Autodesk Fusion 360 part; units mm, degrees
sketch "Skizze1" plane through (0, 0, 0) normal (0, 1, 0) x (1, 0, 0)
  circle A0 centre (0, 0) radius 71.7
  circle A1 centre (0, 0) radius 68.7
  circle A2 centre (0, 0) radius 25
  circle A3 centre (0, 44) radius 13.5
  circle A4 centre (-38.1051, 22) radius 13.5
  circle A5 centre (-38.1051, -22) radius 13.5
  circle A6 centre (0, -44) radius 13.5
  circle A7 centre (38.1051, -22) radius 13.5
  circle A8 centre (38.1051, 22) radius 13.5
  dimension "d2" = 143.4
  dimension "d3" = 3
  dimension "d4" = 50
  dimension "d11" = 27
  dimension "d13" = 360
  dimension "d17" = 44
  dimension "d25" = 44
extrude "Extrusion1" add sketch "Skizze1" along normal blind 2 contours A1 | A3 | A4 | A5 | A6 | A7 | A8 makes body 1
extrude "Extrusion2" add sketch "Skizze1" against normal blind 1 contours A0 | A1 | A2 | A3 | A4 | A5 | A6 | A7 | A8 bodies 1
extrude "Extrusion3" add sketch "Skizze1" along normal blind 60 contours A0 bodies 1
extrude "Extrusion4" cut sketch "Skizze1" against normal blind 2 from surface at 2 contours A3 | A4 | A5 | A6 | A7 | A8 bodies 1
sketch "Skizze2" plane through (0, 60, 0) normal (0, 1, 0) x (-1, 0, 0)
  circle A0 centre (0, 0) radius 68.7
  circle A1 centre (0, 0) radius 71.7
  circle A2 centre (0, 0) radius 68.3
  circle A3 centre (0, 0) radius 63.7
  dimension "d19" = -0.4
  dimension "d22" = -5
extrude "Extrusion5" add sketch "Skizze2" along normal blind 4 separate body contours A0 | A1 | A2 | A3 makes body 2
extrude "Extrusion6" add sketch "Skizze2" against normal blind 5 contours A2 bodies 2
sketch "Skizze3" plane through (0, -1, 0) normal (0, -1, 0) x (1, 0, 0)
  circle A0 centre (0, 0) radius 71.7
  circle A1 centre (0, 0) radius 75
  dimension "d26" = 150
extrude "Extrusion7" add sketch "Skizze3" along normal blind 5 contours A0 | A1 bodies 1
extrude "Extrusion8" cut 7 faces at (36.4978, 0, -25.6989) (3.6941, 0, -49.6839) (-6.7759, 0, 1.242) (-46.8549, 0, -23.9971) (-34.6344, 0, 25.418) (-1.9803, 0, 52.6763) (42.9135, 0, 25.5182) along direction (0, -1, 0) blind 5 on bodies 1 bodies 1
extrude "Extrusion9" cut 1 faces at (26.9574, 2, -46.6916) along direction (0, -1, 0) blind 5 on bodies 1 bodies 1
move_face "Flächen versetzen1" offset -1 1 faces at (68.6146, 39, 3.4244) on bodies 1
extrude "Extrusion10" cut 1 faces at (-22.538, 60, -67.176) along direction (0, -1, 0) blind 13 on bodies 1 bodies 1
hidden bodies 2
equation "Durchmesser = Plexidurchmesser - 3 mm - 3 mm - 0.6 mm"
equation "d2 = Durchmesser"
equation "Plexidurchmesser = 150 mm"
The listing builds one solid part. Answer for the finished solid, in the listing's coordinates (mm). A direction names the side the tool comes from. Give positions to 0.01 mm unless a question says otherwise; leave off trailing zeros. Write each loop counter-clockwise with the first axis right and the second up, starting at its lowest first coordinate (ties: lowest second). Pieces come first, ordered by that corner, then holes. Notation, with made-up numbers: (72.5, 87.5) -> (101.5, 87.5) arc R13 cw to (101.5, 112.5) -> close; hole circle Ø9 at (52.25, 68.25). An arc over 180 degrees is marked (long way). Use one line per item in the form item = value.
1) Straight lines are drawn through the part: probe 1 along Z at (x, y) = (0, -4); probe 2 along Z at (x, y) = (1.5, 41.5); probe 3 along X at (y, z) = (22.5, -43) (3 decimals). For each, find the intervals that lie inside material, in ascending order.
Result:
probe_1 = -75 to -57.5, -30.5 to -25, 25 to 30.5, 57.5 to 75
probe_2 = -71.68 to -69.68, 69.68 to 71.68
probe_3 = -57.375 to -54.855, 54.855 to 57.375
2) Section D-D on z = -59.5 is taken. Write down the section's boundary in (x, y), plus the area to 3 significant figures.
Result:
outline = (-45.66, -6) -> (45.66, -6) -> (45.66, -1) -> (40.01, -1) -> (40.01, 47) -> (36.3, 47) -> (36.3, -3) -> (-36.3, -3) -> (-36.3, 47) -> (-40.01, 47) -> (-40.01, -1) -> (-45.66, -1) -> close
area = 667 mm²
3) A tool of negligible diameter and unlimited length cuts with its end or side. For faces 4 (the cylindrical face through (-48.82, -3.99, 30.21)), 5 (the flat face through (-59, 47, -38)), from which of +Z, -Z, +X, -X, +Y, -Y can it reach the whole face along a straight path? Write none if from no direction.
Result:
face_4 = +Y
face_5 = +Z, -Z, +X, -X, +Y
4) Section B-B on x = 0 is taken. Write down the section's boundary in (y, z).
Result:
outline = (-6, -75) -> (-1, -75) -> (-1, -71.7) -> (47, -71.7) -> (47, -69.7) -> (-3, -69.7) -> (-3, -57.5) -> (-5, -57.5) -> (-5, -30.5) -> (-3, -30.5) -> (-3, -25) -> (-5, -25) -> (-5, 25) -> (-3, 25) -> (-3, 30.5) -> (-5, 30.5) -> (-5, 57.5) -> (-3, 57.5) -> (-3, 69.7) -> (47, 69.7) -> (47, 71.7) -> (-1, 71.7) -> (-1, 75) -> (-6, 75) -> close
5) Section A-A on z = 0 is taken. Write down the section's boundary in (x, y).
Result:
outline = (-75, -6) -> (75, -6) -> (75, -1) -> (71.7, -1) -> (71.7, 47) -> (69.7, 47) -> (69.7, -3) -> (25, -3) -> (25, -5) -> (-25, -5) -> (-25, -3) -> (-69.7, -3) -> (-69.7, 47) -> (-71.7, 47) -> (-71.7, -1) -> (-75, -1) -> close
6) For a pull along X with two mould halves and no side action, classify faces 1 (the cylindrical face through (-9.764, -3.465, -74.362)), 2 (the cylindrical face through (23.846, -4.014, 7.509)), 3 (the flat face through (-1, -6, 1)) as +X half, -X half, draft (parallel to the pull), parting line (faces both ways), or undercut.
Result:
face_1 = parting line
face_2 = undercut
face_3 = draft
7) Section C-C on y = 13.5 is taken. Write down the section's boundary in (x, z), plus the area to 3 significant figures.
Result:
outline = circle Ø143.4 at (0, 0); hole circle Ø139.4 at (0, 0)
area = 888 mm²
8) Each of these flat-tipped pins is pushed along its axis until it touches: P1, Ø6, axis at y = 20, z = 21, coming from the -X side; P2, Ø12, axis at y = 19, z = -18.5, coming from the +X side; P3, Ø3, axis at x = 15.5, z = -14.5, coming from the +Y side. Where does it stop, or does it pass through?
Result:
P1 = -69.4
P2 = 70.6
P3 = -5
